Design review of the part built by this model. Coordinates are the model's own, in mm. Give positions to 0.01 mm unless a question says otherwise; leave off trailing zeros. Write each loop counter-clockwise with the first axis right and the second up, starting at its lowest first coordinate (ties: lowest second). Pieces come first, ordered by that corner, then holes. Notation, with made-up numbers: (55, 48.25) -> (80, 48.25) arc R11 ccw to (80, 63.25) -> close; hole circle Ø7 at (1, 78.5). An arc over 180 degrees is marked (long way). Return JSON: item names as keys, results as strings. Group by question number.
from build123d import *

# Parameters (mm, degrees)
ESBO_O1_R          = 31
ESBO_O1_R_2        = 4.5
FLANGE_BASE1_DEPTH = 2


# Sheet-metal steps are written as plain solids
with BuildPart() as part:
    # Esboço1 → Flange-base1 (new body)
    with BuildSketch(Plane(origin=(0, 0, 0), x_dir=(1, 0, 0), z_dir=(0, 1, 0))):
        with BuildLine():
            Line((-22.09063369, 43.737900077), (-48.92344942, -2.737900077))
            ThreePointArc((-48.92344942, -2.737900077), (-42.435244785, -24.5), (-26.83281573, -41))
            Line((-26.83281573, -41), (26.83281573, -41))
            ThreePointArc((26.83281573, -41), (42.435244785, -24.5), (48.92344942, -2.737900077))
            Line((48.92344942, -2.737900077), (22.09063369, 43.737900077))
            ThreePointArc((22.09063369, 43.737900077), (0, 49), (-22.09063369, 43.737900077))
        make_face()
        with Locations(Location((0, 0, 0), (0, 0, 270))):
            Circle(ESBO_O1_R, mode=Mode.SUBTRACT)
        with Locations(Location((0, 39.5, 0), (0, 0, 270))):
            Circle(ESBO_O1_R_2, mode=Mode.SUBTRACT)
        with Locations(Location((34.208003449, -19.75, 0), (0, 0, 270))):
            Circle(ESBO_O1_R_2, mode=Mode.SUBTRACT)
        with Locations(Location((-34.208003449, -19.75, 0), (0, 0, 270))):
            Circle(ESBO_O1_R_2, mode=Mode.SUBTRACT)
    extrude(amount=-FLANGE_BASE1_DEPTH)


solid = part.part
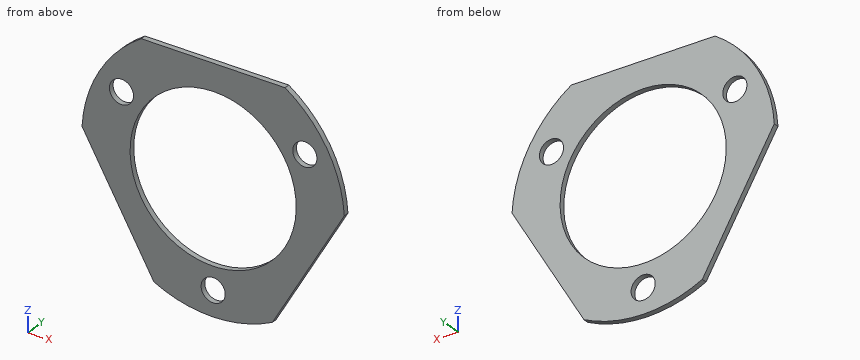
Q1. Take a section at C-C, the plane y = -1.4. Give the boundary of the cut face in (x, z).
Q2. Take a section at D-D, the plane z = 19.75. Give the boundary of the cut face in (x, y), plus the area to 3 significant figures.
Q3. Take a section at A-A, the plane x = 0. Give the boundary of the cut face in (y, z).
Q4. Take a section at B-B, the plane z = -11. Give the boundary of the cut face in (x, y).
Q5. For L1, parallel to X at y = -1.55, z = 18; L2, parallel to Z at x = 37, y = -0.5; L3, parallel to Z at x = -6, y = -0.4, list the stretches that pass through material, from the lowest coordinate up. Write a range as from..to.
Final values:
{
 "1": {"outline": "(-48.92, 2.74) -> (-22.09, -43.74) arc R49 ccw to (22.09, -43.74) -> (48.92, 2.74) arc R49 ccw to (26.83, 41) -> (-26.83, 41) arc R49 ccw to start; hole circle Ø9 at (-34.21, 19.75); hole circle Ø62 at (0, 0); hole circle Ø9 at (0, -39.5); hole circle Ø9 at (34.21, 19.75)"},
 "2": {"outline": "(-44.84, -2) -> (-38.71, -2) -> (-38.71, 0) -> (-44.84, 0) -> close; (-29.71, -2) -> (-23.89, -2) -> (-23.89, 0) -> (-29.71, 0) -> close; (23.89, -2) -> (29.71, -2) -> (29.71, 0) -> (23.89, 0) -> close; (38.71, -2) -> (44.84, -2) -> (44.84, 0) -> (38.71, 0) -> close", "area": "47.8 mm²"},
 "3": {"outline": "(-2, -49) -> (0, -49) -> (0, -44) -> (-2, -44) -> close; (-2, -35) -> (0, -35) -> (0, -31) -> (-2, -31) -> close; (-2, 31) -> (0, 31) -> (0, 41) -> (-2, 41) -> close"},
 "4": {"outline": "(-40.99, -2) -> (-28.98, -2) -> (-28.98, 0) -> (-40.99, 0) -> close; (28.98, -2) -> (40.99, -2) -> (40.99, 0) -> (28.98, 0) -> close"},
 "5": {"L1": "x = -45.57..-38.35, -30.06..-25.24, 25.24..30.06, 38.35..45.57", "L2": "z = -17.91..16.22, 23.28..32.12", "L3": "z = -48.63..-30.41, 30.41..41"}
}
